Geometry check sheet. Reference: the model listing, model coordinates, mm. Face numbers are marked on the shaded views. Give positions to 0.01 mm unless a question says otherwise; leave off trailing zeros. Write each loop counter-clockwise with the first axis right and the second up, starting at its lowest first coordinate (ties: lowest second). Pieces come first, ordered by that corner, then holes. Notation, with made-up numbers: (76, 13.5) -> (127, 13.5) arc R14 cw to (127, 23.5) -> close; hole circle Ø10 at (-32, 20.25). An arc over 180 degrees is marked (long way). One line per item, written item: value.
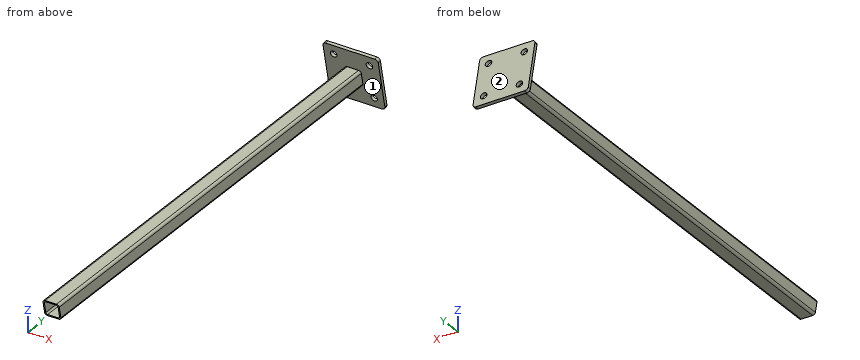
from build123d import *

# Parameters (mm, degrees)
F0_W     = 31.75
F0_H     = 31.75
F0_W_2   = 26.924
F0_H_2   = 26.924
F1_DEPTH = 457.2
F2_R     = 4.7752
F3_R     = 3.175
F5_DEPTH = 31.751
F6_R     = 6.35
F7_DEPTH = 6.35


with BuildPart() as f1:
    # F0 (on Front) → F1 (new body, symmetric)
    with BuildSketch(Plane.XZ):
        Rectangle(F0_W, F0_H)
        Rectangle(F0_W_2, F0_H_2, mode=Mode.SUBTRACT)
    extrude(amount=F1_DEPTH, both=True)

    # F2
    f2_edges = [f1.edges().sort_by_distance(p)[0] for p in [
        (15.875, 0, -15.875),
        (-15.875, 0, -15.875),
        (-15.875, 0, 15.875),
        (15.875, 0, 15.875),
    ]]
    fillet(f2_edges, radius=F2_R)

    # F3
    f3_edges = [f1.edges().sort_by_distance(p)[0] for p in [
        (-13.462, 0, 13.462),
        (13.462, 0, 13.462),
        (-13.462, 0, -13.462),
        (13.462, 0, -13.462),
    ]]
    fillet(f3_edges, radius=F3_R)

    # F4 (on face) → F5 (cut, through all)
    with BuildSketch(Plane.YZ.offset(15.875)):
        Polygon((-450.451329167, -15.875), (-457.2, 15.875), (-457.2, -15.875), align=None)
        Polygon((457.2, 15.875), (450.451329167, 15.875), (457.2, -15.875), align=None)
    extrude(amount=-F5_DEPTH, mode=Mode.SUBTRACT)

    # F6 (on face) → F7 (join)
    with BuildSketch(Plane(origin=(0, 434.2080195127, 92.2937636772), x_dir=(-1, 0, 0), z_dir=(0, 0.9781476007, 0.2079116908))):
        with BuildLine():
            Line((-47.625, -148.33066126), (47.625, -148.33066126))
            ThreePointArc((47.625, -148.33066126), (52.1151280605, -146.4707893206), (53.975, -141.98066126))
            Line((53.975, -141.98066126), (53.975, -46.73066126))
            ThreePointArc((53.975, -46.73066126), (52.1151280605, -42.2405331995), (47.625, -40.38066126))
            Line((47.625, -40.38066126), (-47.625, -40.38066126))
            ThreePointArc((-47.625, -40.38066126), (-52.1151280605, -42.2405331995), (-53.975, -46.73066126))
            Line((-53.975, -46.73066126), (-53.975, -141.98066126))
            ThreePointArc((-53.975, -141.98066126), (-52.1151280605, -146.4707893206), (-47.625, -148.33066126))
        make_face()
        with Locations((-34.925, -129.28066126)):
            Circle(F6_R, mode=Mode.SUBTRACT)
        with Locations((34.925, -129.28066126)):
            Circle(F6_R, mode=Mode.SUBTRACT)
        with Locations((-34.925, -59.43066126)):
            Circle(F6_R, mode=Mode.SUBTRACT)
        with Locations((34.925, -59.43066126)):
            Circle(F6_R, mode=Mode.SUBTRACT)
    extrude(amount=F7_DEPTH)


solid = f1.part
1) Sectioned sample at A-A on y = -236. Record the cut outline in (x, z) (3 decimals).
Verdict:
outline: (-15.875, -11.1) arc R4.775 ccw to (-11.1, -15.875) -> (11.1, -15.875) arc R4.775 ccw to (15.875, -11.1) -> (15.875, 11.1) arc R4.775 ccw to (11.1, 15.875) -> (-11.1, 15.875) arc R4.775 ccw to (-15.875, 11.1) -> close; hole (-13.462, -10.287) arc R3.175 ccw to (-10.287, -13.462) -> (10.287, -13.462) arc R3.175 ccw to (13.462, -10.287) -> (13.462, 10.287) arc R3.175 ccw to (10.287, 13.462) -> (-10.287, 13.462) arc R3.175 ccw to (-13.462, 10.287) -> close
2) Scan lines: probe 1 along Z at (x, y) = (8.5, 199) (3 decimals); probe 2 along Y at (x, z) = (24.5, -20). Record each from-to range of solid material in increasing order.
Verdict:
probe 1: -15.875 to -13.462, 13.462 to 15.875
probe 2: 458.08 to 464.57
3) Depth check by flat-ended pin: pin 1 Ø6 at (y, z) = (166.5, 3) entering from -X (3 decimals); pin 2 Ø2 at (x, z) = (22.5, -26.5) entering from -Y; pin 3 Ø1.5 at (y, z) = (369, -18) entering from -X; pin 4 Ø10 at (x, z) = (21.5, -14) entering from +Y. Enter the tip coordinate at first touch or a pass-through.
Verdict:
pin 1: x = -15.875
pin 2: y = 459.25
pin 3: through
pin 4: y = 464.36
4) Sectioned sample at B-B on x = 2.5. Record the cut outline in (y, z) (3 decimals).
Verdict:
outline: (-457.2, 15.875) -> (-456.687, 13.462) -> (450.964, 13.462) -> (456.687, -13.462) -> (-450.964, -13.462) -> (-450.451, -15.875) -> (457.2, -15.875) -> (465.048, -52.796) -> (471.259, -51.475) -> (448.815, 54.116) -> (442.604, 52.796) -> (450.451, 15.875) -> close
5) Mould release check, pull along Z, two halves, no side actions. Record for the marked faces 1 and 2: released by +Z, released by -Z, zero draft, split by the parting line, or undercut.
Verdict:
face 1: undercut
face 2: released by +Z
